Geometry: final body of the model. Coordinates: model frame, mm. Face numbers are marked on the shaded views. A direction names the side the tool comes from. Give positions to 0.01 mm unless a question says otherwise; leave off trailing zeros. Write each loop counter-clockwise with the first axis right and the second up, starting at its lowest first coordinate (ties: lowest second). Pieces come first, ordered by that corner, then holes. Notation, with made-up numbers: (-30.5, -39.75) - (-22.5, -39.75) arc R14 ccw to (-22.5, -30.75) - close; hole circle Ø7 at (10.5, 43.5). An arc over 180 degrees is marked (long way). Return JSON: item names as keys, results as strings.
from build123d import *

# Parameters (mm, degrees)
SKETCH1_R               = 0.5
BOSS_EXTRUDE1_DEPTH     = 2.25
CUT_EXTRUDE3_DEPTH      = 1
CUT_EXTRUDE4_DEPTH      = 1.25
BOSS_EXTRUDE2_DEPTH     = 2.25
SKETCH7_R               = 1
BOSS_EXTRUDE3_DEPTH     = 2
SKETCH8_R               = 0.5
CUT_EXTRUDE5_DEPTH      = 3
M3_5_TAPPED_HOLE1_D     = 2.9
M3_5_TAPPED_HOLE1_DEPTH = 2
M3_5_TAPPED_HOLE1_TIP   = 0.871247898


with BuildPart() as part:
    # Sketch1 → Boss-Extrude1 (new body)
    with BuildSketch(Plane(origin=(0, 0, -0.343889451), x_dir=(1, 0, 0), z_dir=(0, 1, 0))):
        with BuildLine():
            Line((0, -0.009375659), (6, -0.009375659))
            Line((6, -0.009375659), (10, -3.259375659))
            ThreePointArc((10, -3.259375659), (10.670843802, -4.509375659), (10, -5.759375659))
            Line((10, -5.759375659), (6, -9.009375659))
            Line((6, -9.009375659), (0, -9.009375659))
            Line((0, -9.009375659), (-4, -5.759375659))
            ThreePointArc((-4, -5.759375659), (-4.670843802, -4.509375659), (-4, -3.259375659))
            Line((-4, -3.259375659), (0, -0.009375659))
        make_face()
        with Locations((-3.170843802, -4.509375659)):
            Circle(SKETCH1_R, mode=Mode.SUBTRACT)
    extrude(amount=BOSS_EXTRUDE1_DEPTH)

    # Sketch4 → Cut-Extrude3 (cut)
    with BuildSketch(Plane.XZ):
        with BuildLine():
            Line((-4.288877791, 5.165486209), (-0.670843802, 5.165486209))
            Line((-0.670843802, 5.165486209), (-0.670843802, 3.165486209))
            Line((-0.670843802, 3.165486209), (-4.288877791, 3.165486209))
            ThreePointArc((-4.288877791, 3.165486209), (-4.670843802, 4.165486209), (-4.288877791, 5.165486209))
        make_face()
    extrude(amount=-CUT_EXTRUDE3_DEPTH, mode=Mode.SUBTRACT)

    # Sketch5 → Cut-Extrude4 (cut)
    with BuildSketch(Plane(origin=(0, 0, 0), x_dir=(-1, 0, 0), z_dir=(0, -1, 0))):
        with BuildLine():
            Line((0.170843802, -7.665486209), (-6.170843802, -7.665486209))
            ThreePointArc((-6.170843802, -7.665486209), (-6.524397193, -7.519039599), (-6.670843802, -7.165486209))
            Line((-6.670843802, -7.165486209), (-6.670843802, -1.165486209))
            ThreePointArc((-6.670843802, -1.165486209), (-6.524397193, -0.811932818), (-6.170843802, -0.665486209))
            Line((-6.170843802, -0.665486209), (0.170843802, -0.665486209))
            ThreePointArc((0.170843802, -0.665486209), (0.524397193, -0.811932818), (0.670843802, -1.165486209))
            Line((0.670843802, -1.165486209), (0.670843802, -7.165486209))
            ThreePointArc((0.670843802, -7.165486209), (0.524397193, -7.519039599), (0.170843802, -7.665486209))
        make_face()
    extrude(amount=-CUT_EXTRUDE4_DEPTH, mode=Mode.SUBTRACT)

    # Sketch6 → Boss-Extrude2 (add)
    with BuildSketch(Plane(origin=(0, 2.25, 0), x_dir=(1, 0, 0), z_dir=(0, 1, 0))):
        Polygon((0.593843358, -3.915486209), (3.093843358, -3.915486209), (3.093843358, -1.665486209), (4.093843358, -1.665486209), (4.093843358, -6.665486209), (3.093843358, -6.665486209), (3.093843358, -4.415486209), (0.593843358, -4.415486209), align=None)
    extrude(amount=BOSS_EXTRUDE2_DEPTH)

    # Sketch7 → Boss-Extrude3 (add)
    with BuildSketch(Plane(origin=(0, 4.5, 0), x_dir=(1, 0, 0), z_dir=(0, 1, 0))):
        with BuildLine():
            Line((-1.906156642, -1.665486209), (-1.906156642, -2.656110549))
            ThreePointArc((-1.906156642, -2.656110549), (-0.406156642, -4.156110549), (-1.906156642, -5.656110549))
            Line((-1.906156642, -5.656110549), (-1.906156642, -6.665486209))
            Line((-1.906156642, -6.665486209), (8.093843358, -6.665486209))
            ThreePointArc((8.093843358, -6.665486209), (10.593843358, -4.165486209), (8.093843358, -1.665486209))
            Line((8.093843358, -1.665486209), (-1.906156642, -1.665486209))
        make_face()
        with Locations((8.093843358, -4.165486209)):
            Circle(SKETCH7_R, mode=Mode.SUBTRACT)
    extrude(amount=BOSS_EXTRUDE3_DEPTH)

    # Sketch8 → Cut-Extrude5 (cut)
    with BuildSketch(Plane(origin=(0, 2.25, 0), x_dir=(1, 0, 0), z_dir=(0, 1, 0))):
        with Locations((8.093843358, -4.165486209)):
            Circle(SKETCH8_R)
    extrude(amount=-CUT_EXTRUDE5_DEPTH, mode=Mode.SUBTRACT)

    # M3.5 Tapped Hole1
    with Locations(Plane(origin=(8.093843358, 6.5, 4.165486209), x_dir=(0, 0, 1), z_dir=(0, 1, 0))):
        with Locations((0, 0)):
            Hole(M3_5_TAPPED_HOLE1_D / 2, depth=M3_5_TAPPED_HOLE1_DEPTH)
            with Locations((0, 0, -(M3_5_TAPPED_HOLE1_DEPTH + M3_5_TAPPED_HOLE1_TIP / 2))):  # 118° drill point
                Cone(0, M3_5_TAPPED_HOLE1_D / 2, M3_5_TAPPED_HOLE1_TIP, mode=Mode.SUBTRACT)


solid = part.part
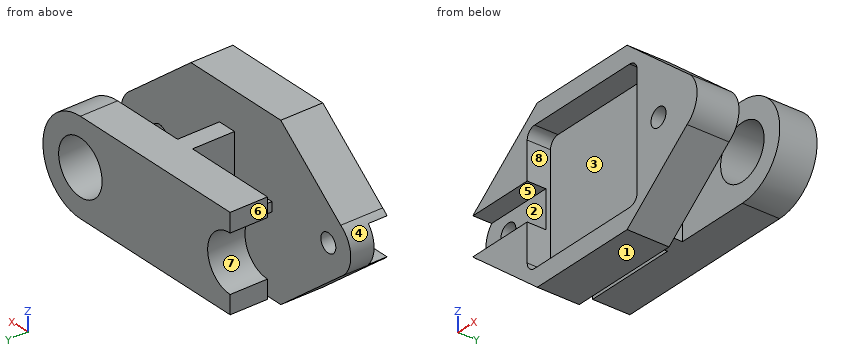
Q1. Section query A-A, the plane x = 9. Return the cut outline in (y, z).
Answer key:
{"outline": "(0, 2.1) - (2.25, 2.1) - (2.25, 6.23) - (0, 6.23) - close; (4.5, 1.84) - (6.5, 1.84) - (6.5, 3.03) - (4.5, 3.03) - close; (4.5, 5.3) - (6.5, 5.3) - (6.5, 6.5) - (4.5, 6.5) - close"}
Q2. Section query D-D, the plane y = 0.75. Return the cut outline in (x, z).
Answer key:
{"outline": "(-4.29, 3.17) arc R1.5 ccw to (-4, 2.92) - (0, -0.33) - (6, -0.33) - (10, 2.92) arc R1.5 ccw to (10, 5.42) - (6, 8.67) - (0, 8.67) - (-4, 5.42) arc R1.5 ccw to (-4.29, 5.17) - (-0.67, 5.17) - (-0.67, 7.17) arc R0.5 cw to (-0.17, 7.67) - (6.17, 7.67) arc R0.5 cw to (6.67, 7.17) - (6.67, 1.17) arc R0.5 cw to (6.17, 0.67) - (-0.17, 0.67) arc R0.5 cw to (-0.67, 1.17) - (-0.67, 3.17) - close; hole circle Ø1 at (8.09, 4.17)"}
Q3. Section query C-C, the plane x = 2.5. Return the cut outline in (y, z), plus the area to 3 significant figures.
Answer key:
{"outline": "(0, -0.33) - (2.25, -0.33) - (2.25, 3.92) - (4.5, 3.92) - (4.5, 1.67) - (6.5, 1.67) - (6.5, 6.67) - (4.5, 6.67) - (4.5, 4.42) - (2.25, 4.42) - (2.25, 8.67) - (0, 8.67) - (0, 7.67) - (1.25, 7.67) - (1.25, 0.67) - (0, 0.67) - close", "area": "22.6 mm^2"}
Q4. Section query B-B, the plane y = 1.5. Return the cut outline in (x, z).
Answer key:
{"outline": "(-4, 2.92) - (0, -0.33) - (6, -0.33) - (10, 2.92) arc R1.5 ccw to (10, 5.42) - (6, 8.67) - (0, 8.67) - (-4, 5.42) arc R1.5 ccw to start; hole circle Ø1 at (-3.17, 4.17); hole circle Ø1 at (8.09, 4.17)"}
Q5. Material intervals for probe 1 along Y at (x, z) = (4.5, 6); probe 2 along Z at (x, y) = (5.25, 6); probe 3 along Y at (x, z) = (1.5, 1.25), sorted ascending. Write a range as [from, to].
Answer key:
{"probe 1": "y = [1.25, 2.25], [4.5, 6.5]", "probe 2": "z = [1.67, 6.67]", "probe 3": "y = [1.25, 2.25]"}
Q6. Pin query (flat end, axial travel): P1, Ø2.5, axis at y = 3.5, z = 5, coming from the +X side; P2, Ø0.5, axis at y = 5.5, z = 6.5, coming from the -X side; P3, Ø2, axis at x = 1.5, y = 4.5, coming from the -Z side; P4, Ø2.5, axis at x = 6.5, z = 3.5, coming from the -Y side. Return the tip coordinate at first contact, or that it passes through.
Answer key:
{"P1": "stops at x = 10.59", "P2": "stops at x = -1.91", "P3": "stops at z = 1.67", "P4": "stops at y = 0"}
Q7. Mould query, pull axis Z, two halves, no side actions, for the marked faces 1, 2, 3 and 4. Classes: pulls with the +Z half, pulls with the -Z half, needs draft (parallel to the pull), parting line crosses it, or undercut.
Answer key:
{"face 1": "pulls with the -Z half", "face 2": "undercut", "face 3": "undercut", "face 4": "parting line crosses it"}
Q8. Set-up query: the marked faces 5, 6, 7 and 8. Return all of +Z, -Z, +X, -X, +Y, -Y with unobstructed straight access to the full face (end or side cutting, diameter ignored); none if empty.
Answer key:
{"face 5": "-X, -Y", "face 6": "+Z, -Z, -X, +Y", "face 7": "-X, +Y", "face 8": "-Y"}
